Build history of the part. All positions in model axes, mm. A direction names the side the tool comes from. Round coordinates to 2 decimals unless told otherwise and drop trailing zeros. Write each loop counter-clockwise with the first axis right and the second up, starting at its lowest first coordinate (ties: lowest second). Pieces come first, ordered by that corner, then holes. Notation, with made-up numbers: (-22, 68.5) - (-2, 68.5) arc R11 ccw to (-2, 75.5) - close; hole circle Ø2 at (-8, 57.25). An arc over 180 degrees is marked (long way). Write each question's results on one line, items separated by ' | '.
from build123d import *

# Parameters (mm, degrees)
SKETCH_1_W          = 59
SKETCH_1_H          = 41
EXTRUDE_1_DEPTH     = 25
SKETCH_2_R          = 10.5
EXTRUDE_2_DEPTH     = 5
SKETCH_5_R          = 5
EXTRUDE_3_DEPTH     = 1
SKETCH_6_W          = 10
SKETCH_6_H          = 22
CUT_EXTRUDE_1_DEPTH = 1


with BuildPart() as part:
    # Эскиз1 → Бобышка-Вытянуть1 (new body)
    with BuildSketch(Plane.XY):
        Rectangle(SKETCH_1_W, SKETCH_1_H)
    extrude(amount=EXTRUDE_1_DEPTH)

    # Эскиз2 → Бобышка-Вытянуть2 (add)
    with BuildSketch(Plane.XY.offset(25)):
        with Locations((13.9, 5)):
            Circle(SKETCH_2_R)
    extrude(amount=EXTRUDE_2_DEPTH)

    # Эскиз5 → Бобышка-Вытянуть3 (add)
    with BuildSketch(Plane.XY.offset(25)):
        with Locations((-17.5, 7.5)):
            Circle(SKETCH_5_R)
    extrude(amount=EXTRUDE_3_DEPTH)

    # Эскиз6 → Вырез-Вытянуть1 (cut)
    with BuildSketch(Plane(origin=(29.5, 0, 0), x_dir=(0, 0, -1), z_dir=(1, 0, 0))):
        with Locations((-8, 1.5)):
            Rectangle(SKETCH_6_W, SKETCH_6_H)
    extrude(amount=-CUT_EXTRUDE_1_DEPTH, mode=Mode.SUBTRACT)


solid = part.part
(1) Slice it at D-D, the plane y = -4. Write the cut outline in (x, z), and give its area (3 significant figures).
Worked answers:
outline: (-29.5, 0) - (29.5, 0) - (29.5, 3) - (28.5, 3) - (28.5, 13) - (29.5, 13) - (29.5, 25) - (19.31, 25) - (19.31, 30) - (8.49, 30) - (8.49, 25) - (-29.5, 25) - close | area: 1,520 mm2
(2) Slice it at A-A, the plane x = -17.5. Write the cut outline in (y, z).
Worked answers:
outline: (-20.5, 0) - (20.5, 0) - (20.5, 25) - (12.5, 25) - (12.5, 26) - (2.5, 26) - (2.5, 25) - (-20.5, 25) - close
(3) Tool access for faces 4 (the flat face through (28.5, 2, 8)), 5 (the flat face through (14, 5, 30)), 6 (the flat face through (-18, 8, 26)), 7 (the cylindrical face through (11.62, -5.25, 27.46)): list every direction of +Z, -Z, +X, -X, +Y, -Y with a clear straight run to the whole face (end or side of a thin tool).
Worked answers:
face 4: +X | face 5: +Z, +X, -X, +Y, -Y | face 6: +Z, -X, +Y, -Y | face 7: +Z
(4) Slice it at C-C, the plane x = 13.9. Write the cut outline in (y, z), and give its area (3 significant figures).
Worked answers:
outline: (-20.5, 0) - (20.5, 0) - (20.5, 25) - (15.5, 25) - (15.5, 30) - (-5.5, 30) - (-5.5, 25) - (-20.5, 25) - close | area: 1,130 mm2
(5) Drill centre lines: probe 1 along Z at (x, y) = (-16, 13); probe 2 along X at (y, z) = (10.5, 11); probe 3 along Z at (x, y) = (-22, 9.5). Where is each one in solid material? Low to high. Write a range as [from, to].
Worked answers:
probe 1: z = [0, 25] | probe 2: x = [-29.5, 28.5] | probe 3: z = [0, 26]
(6) Two-plate mould, pull along X, no slides. Class faces 1 (the flat face through (29.5, 0, 15)), 2 (the flat face through (0, 20.5, 12)), 3 (the cylindrical face through (-21.185, 10.879, 25.493)): released by +X, released by -X, zero draft, split by the parting line, or undercut.
Worked answers:
face 1: released by +X | face 2: zero draft | face 3: undercut
(7) Flat gauge pins, fed straight in: pin 1 Ø8 at (x, y) = (-20, 9.5) entering from +Z; pin 2 Ø5 at (x, y) = (-3, 12) entering from +Z. Where does each tip first touch, or does it go through?
Worked answers:
pin 1: stops at z = 26 | pin 2: stops at z = 25
(8) Slice it at B-B, the plane y = 7.5. Write the cut outline in (x, z).
Worked answers:
outline: (-29.5, 0) - (29.5, 0) - (29.5, 3) - (28.5, 3) - (28.5, 13) - (29.5, 13) - (29.5, 25) - (24.1, 25) - (24.1, 30) - (3.7, 30) - (3.7, 25) - (-12.5, 25) - (-12.5, 26) - (-22.5, 26) - (-22.5, 25) - (-29.5, 25) - close
